Work out the finished part from the listing and answer in its coordinate system (mm). Face numbers are marked on the shaded views. Round coordinates to 2 decimals unless told otherwise and drop trailing zeros. Write each loop counter-clockwise with the first axis right and the second up, starting at its lowest first coordinate (ties: lowest second). Pieces come first, ordered by that corner, then holes. Notation, with made-up numbers: (40, -2) -> (81, -2) arc R25 ccw to (81, 26) -> close; hole circle Ø3 at (86, 14.25). An arc over 180 degrees is marked (long way). Answer as a JSON object with one key per item and string values. Group by question number.
from build123d import *

# Parameters (mm, degrees)
SKETCH1_W           = 44
SKETCH1_H           = 44
SKETCH1_W_2         = 38
SKETCH1_H_2         = 38
BOSS_EXTRUDE1_DEPTH = 25
SKETCH2_W           = 57
SKETCH2_H           = 57
BOSS_EXTRUDE2_DEPTH = 10
SKETCH3_W           = 51.5
SKETCH3_H           = 51.5
SKETCH3_W_2         = 44
SKETCH3_H_2         = 44
CUT_EXTRUDE1_DEPTH  = 4
FILLET1_R           = 2


with BuildPart() as part:
    # Sketch1 → Boss-Extrude1 (new body)
    with BuildSketch(Plane(origin=(0, 0, 0), x_dir=(1, 0, 0), z_dir=(0, 1, 0))):
        Rectangle(SKETCH1_W, SKETCH1_H)
        Rectangle(SKETCH1_W_2, SKETCH1_H_2, mode=Mode.SUBTRACT)
    extrude(amount=BOSS_EXTRUDE1_DEPTH)

    # Sketch2 → Boss-Extrude2 (add)
    with BuildSketch(Plane(origin=(0, 25, 0), x_dir=(1, 0, 0), z_dir=(0, 1, 0))):
        Rectangle(SKETCH2_W, SKETCH2_H)
    extrude(amount=BOSS_EXTRUDE2_DEPTH)

    # Sketch3 → Cut-Extrude1 (cut)
    with BuildSketch(Plane.XZ.offset(-25)):
        Rectangle(SKETCH3_W, SKETCH3_H)
        Rectangle(SKETCH3_W_2, SKETCH3_H_2, mode=Mode.SUBTRACT)
    extrude(amount=-CUT_EXTRUDE1_DEPTH, mode=Mode.SUBTRACT)

    # Fillet1
    fillet1_edges = [part.edges().sort_by_distance(p)[0] for p in [
        (28.5, 25, 0),
        (28.5, 30, 28.5),
        (0, 25, -28.5),
        (28.5, 30, -28.5),
        (-28.5, 25, 0),
        (-28.5, 30, -28.5),
        (0, 25, 28.5),
        (-28.5, 30, 28.5),
        (28.5, 35, 0),
        (0, 35, -28.5),
        (-28.5, 35, 0),
        (0, 35, 28.5),
        (22, 14.5, 22),
        (-22, 14.5, 22),
        (-22, 14.5, -22),
        (22, 14.5, -22),
    ]]
    fillet(fillet1_edges, radius=FILLET1_R)


solid = part.part
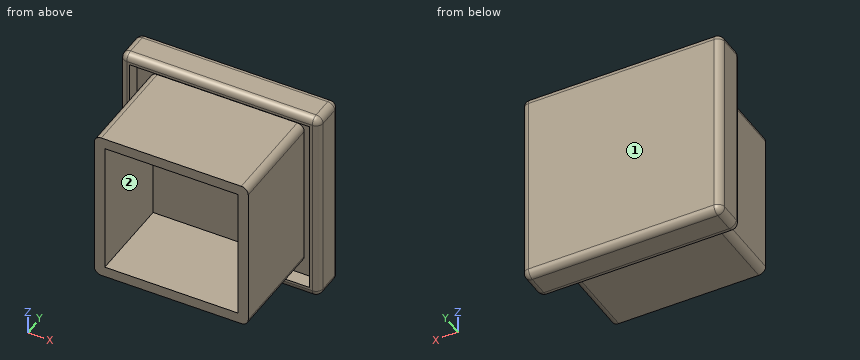
1) A cutting plane is placed at A-A on y = 28. Determine the outline of the cut face in (x, z), plus the area to 3 significant figures.
2) Straight lines are drawn through the part: L1, parallel to X at y = 23.5, z = 16.5; L2, parallel to Z at x = -7, y = 28.5. For each, find the intervals that lie inside material, in ascending order.
3) Each of these flat-tipped pins is pushed along its axis until it touches: P1, Ø15.5, axis at x = 0.5, z = -5.5, coming from the -Y side; P2, Ø12, axis at x = 18, y = 12, coming from the -Z side; P3, Ø14.5, axis at x = 5.5, y = 12, coming from the +Z side. Where does it stop, or does it pass through?
4) For a pull along Z with two mould halves and no side action, classify the marked faces 1 and 2 as released by +Z, released by -Z, zero draft, split by the parting line, or undercut.
5) A cutting plane is placed at D-D on x = -25. Determine the outline of the cut face in (y, z), plus the area to 3 significant figures.
6) A cutting plane is placed at B-B on y = 8.5. Determine the outline of the cut face in (x, z).
7) A cutting plane is placed at C-C on z = -24. Determine the outline of the cut face in (x, y).
Established:
{
 "1": {"outline": "(-28.5, -26.5) arc R2 ccw to (-26.5, -28.5) -> (26.5, -28.5) arc R2 ccw to (28.5, -26.5) -> (28.5, 26.5) arc R2 ccw to (26.5, 28.5) -> (-26.5, 28.5) arc R2 ccw to (-28.5, 26.5) -> close; (-22, -20) arc R2 ccw to (-20, -22) -> (20, -22) arc R2 ccw to (22, -20) -> (22, 20) arc R2 ccw to (20, 22) -> (-20, 22) arc R2 ccw to (-22, 20) -> close; hole (-25.75, -25.75) -> (25.75, -25.75) -> (25.75, 25.75) -> (-25.75, 25.75) -> close", "area": "2,530 mm²"},
 "2": {"L1": "x = -22 to -19, 19 to 22", "L2": "z = -28.5 to -25.75, -22 to 22, 25.75 to 28.5"},
 "3": {"P1": "stops at y = 25", "P2": "stops at z = -22", "P3": "stops at z = 22"},
 "4": {"face 1": "zero draft", "face 2": "undercut"},
 "5": {"outline": "(25, -26.5) arc R2 ccw to (27, -28.5) -> (33, -28.5) arc R2 ccw to (35, -26.5) -> (35, 26.5) arc R2 ccw to (33, 28.5) -> (27, 28.5) arc R2 ccw to (25, 26.5) -> (25, 25.75) -> (29, 25.75) -> (29, -25.75) -> (25, -25.75) -> close", "area": "361 mm²"},
 "6": {"outline": "(-22, -20) arc R2 ccw to (-20, -22) -> (20, -22) arc R2 ccw to (22, -20) -> (22, 20) arc R2 ccw to (20, 22) -> (-20, 22) arc R2 ccw to (-22, 20) -> close; hole (-19, -19) -> (19, -19) -> (19, 19) -> (-19, 19) -> close"},
 "7": {"outline": "(-28.5, 27) arc R2 ccw to (-26.5, 25) -> (-25.75, 25) -> (-25.75, 29) -> (25.75, 29) -> (25.75, 25) -> (26.5, 25) arc R2 ccw to (28.5, 27) -> (28.5, 33) arc R2 ccw to (26.5, 35) -> (-26.5, 35) arc R2 ccw to (-28.5, 33) -> close"}
}
